Input: part model. Units: mm. Frame: model coordinates. A direction names the side the tool comes from. Give positions to 0.01 mm unless a question says otherwise; leave off trailing zeros. Loops run counter-clockwise (first coordinate to the right, second up) from the corner with the lowest first, then second, coordinate; pieces in that order, holes last. Notation, with made-up numbers: (17, 64.5) -> (71, 64.5) arc R36 ccw to (71, 98.5) -> close; hole circle Ø11 at (-31.75, 3.25). An arc over 180 degrees is marked (long way). One line per question, with ' | ' between items.
from build123d import *

# Parameters (mm, degrees)
SKETCH2_R               = 14
SKETCH2_R_2             = 10
EXTRUDE1_DEPTH          = 25.5
EXTRUDE2_DEPTH          = 10
SKETCH4_W               = 51
SKETCH4_H               = 51
EXTRUDE3_DEPTH          = 3
SKETCH5_W               = 51
SKETCH5_H               = 51
SKETCH5_W_2             = 43
SKETCH5_H_2             = 43
EXTRUDE4_DEPTH          = 40
SKETCH8_W               = 25
SKETCH8_H               = 20
EXTRUDE8_DEPTH          = 40
SKETCH10_W              = 43
SKETCH10_H              = 43
EXTRUDE10_DEPTH         = 45
SKETCH11_R              = 15
EXTRUDE11_DEPTH         = 5
SKETCH12_W              = 5
SKETCH12_H              = 25
EXTRUDE12_DEPTH         = 5
SKETCH13_R              = 1.5
EXTRUDE13_DEPTH         = 5
SKETCH14_R              = 7.5
EXTRUDE14_DEPTH         = 10
SKETCH15_R              = 12.5
EXTRUDE15_DEPTH         = 30
SKETCH16_R              = 5
EXTRUDE16_DEPTH         = 125
EXTRUDE17_START         = 80.797218397
EXTRUDE17_OUTLINE_R     = 12.5
EXTRUDE17_OUTLINE_R_2   = 11.5
EXTRUDE17_DEPTH         = 3.587847701
EXTRUDE17_START_2       = 86.797218397
EXTRUDE17_2_OUTLINE_R   = 12.5
EXTRUDE17_2_OUTLINE_R_2 = 11.5
EXTRUDE17_2_DEPTH       = 3.587847701
EXTRUDE17_START_3       = 92.797218397
EXTRUDE17_3_OUTLINE_R   = 12.5
EXTRUDE17_3_OUTLINE_R_2 = 11.5
EXTRUDE17_3_DEPTH       = 3.587847701
EXTRUDE17_START_4       = 98.797218397
EXTRUDE17_4_OUTLINE_R   = 12.5
EXTRUDE17_4_OUTLINE_R_2 = 11.5
EXTRUDE17_4_DEPTH       = 3.587847701


# Read off the part's stored shape, not the designer's step: Extrude17
with BuildPart() as part:
    # Sketch2 → Extrude1 (new, symmetric)
    with BuildSketch(Plane.XY):
        Circle(SKETCH2_R)
        Circle(SKETCH2_R_2, mode=Mode.SUBTRACT)
    extrude(amount=EXTRUDE1_DEPTH, both=True)

    # Sketch3 → Extrude2 (add, symmetric)
    with BuildSketch(Plane.XY):
        with BuildLine():
            Line((0, 14), (15, 14))
            Line((15, 14), (15, -14))
            Line((15, -14), (0, -14))
            ThreePointArc((0, -14), (14, 0), (0, 14))
        make_face()
    extrude(amount=EXTRUDE2_DEPTH, both=True)

    # Sketch4 → Extrude3 (add)
    with BuildSketch(Plane(origin=(15, 0, 0), x_dir=(0, 0, -1), z_dir=(1, 0, 0))):
        Rectangle(SKETCH4_W, SKETCH4_H)
    extrude(amount=EXTRUDE3_DEPTH)

    # Sketch5 → Extrude4 (add)
    with BuildSketch(Plane(origin=(18, 0, 0), x_dir=(0, 0, -1), z_dir=(1, 0, 0))):
        Rectangle(SKETCH5_W, SKETCH5_H)
        Rectangle(SKETCH5_W_2, SKETCH5_H_2, mode=Mode.SUBTRACT)
    extrude(amount=EXTRUDE4_DEPTH)

    # Sketch8 → Extrude8 (cut)
    with BuildSketch(Plane(origin=(58, 0, 0), x_dir=(0, 0, -1), z_dir=(1, 0, 0))):
        with Locations((0, -25.5)):
            Rectangle(SKETCH8_W, SKETCH8_H)
    extrude(amount=-EXTRUDE8_DEPTH, mode=Mode.SUBTRACT)

    # Sketch10 → Extrude10 (add)
    with BuildSketch(Plane(origin=(18, 0, 0), x_dir=(0, 0, -1), z_dir=(1, 0, 0))):
        Rectangle(SKETCH10_W, SKETCH10_H)
    extrude(amount=EXTRUDE10_DEPTH)

    # Sketch11 → Extrude11 (add)
    with BuildSketch(Plane(origin=(63, 0, 0), x_dir=(0, 0, -1), z_dir=(1, 0, 0))):
        Circle(SKETCH11_R)
    extrude(amount=EXTRUDE11_DEPTH)

    # Sketch12 → Extrude12 (add)
    with BuildSketch(Plane.XZ.offset(21.5)):
        with Locations((20.5, 0)):
            Rectangle(SKETCH12_W, SKETCH12_H)
    extrude(amount=EXTRUDE12_DEPTH)

    # Sketch13 → Extrude13 (add)
    with BuildSketch(Plane.XZ.offset(26.5)):
        with Locations(Location((20.514171065, 8.5, 0), (0, 0, 270))):
            Circle(SKETCH13_R)
        with Locations(Location((20.514171065, 3.5, 0), (0, 0, 270))):
            Circle(SKETCH13_R)
        with Locations(Location((20.514171065, -3.5, 0), (0, 0, 270))):
            Circle(SKETCH13_R)
        with Locations(Location((20.514171065, -8.5, 0), (0, 0, 270))):
            Circle(SKETCH13_R)
    extrude(amount=EXTRUDE13_DEPTH)

    # Sketch14 → Extrude14 (add)
    with BuildSketch(Plane(origin=(68, 0, 0), x_dir=(0, 0, -1), z_dir=(1, 0, 0))):
        Circle(SKETCH14_R)
    extrude(amount=EXTRUDE14_DEPTH)

    # Sketch15 → Extrude15 (add)
    with BuildSketch(Plane(origin=(78, 0, 0), x_dir=(0, 0, -1), z_dir=(1, 0, 0))):
        Circle(SKETCH15_R)
    extrude(amount=EXTRUDE15_DEPTH)

    # Sketch16 → Extrude16 (add)
    with BuildSketch(Plane(origin=(108, 0, 0), x_dir=(0, 0, -1), z_dir=(1, 0, 0))):
        Circle(SKETCH16_R)
    extrude(amount=EXTRUDE16_DEPTH)

    # Extrude17 outline → Extrude17 (cut)
    with BuildSketch(Plane.YZ.offset(EXTRUDE17_START)):
        Circle(EXTRUDE17_OUTLINE_R)
        Circle(EXTRUDE17_OUTLINE_R_2, mode=Mode.SUBTRACT)
    extrude(amount=EXTRUDE17_DEPTH, mode=Mode.SUBTRACT)

    # Extrude17 2 outline → Extrude17 2 (cut)
    with BuildSketch(Plane.YZ.offset(EXTRUDE17_START_2)):
        Circle(EXTRUDE17_2_OUTLINE_R)
        Circle(EXTRUDE17_2_OUTLINE_R_2, mode=Mode.SUBTRACT)
    extrude(amount=EXTRUDE17_2_DEPTH, mode=Mode.SUBTRACT)

    # Extrude17 3 outline → Extrude17 3 (cut)
    with BuildSketch(Plane.YZ.offset(EXTRUDE17_START_3)):
        Circle(EXTRUDE17_3_OUTLINE_R)
        Circle(EXTRUDE17_3_OUTLINE_R_2, mode=Mode.SUBTRACT)
    extrude(amount=EXTRUDE17_3_DEPTH, mode=Mode.SUBTRACT)

    # Extrude17 4 outline → Extrude17 4 (cut)
    with BuildSketch(Plane.YZ.offset(EXTRUDE17_START_4)):
        Circle(EXTRUDE17_4_OUTLINE_R)
        Circle(EXTRUDE17_4_OUTLINE_R_2, mode=Mode.SUBTRACT)
    extrude(amount=EXTRUDE17_4_DEPTH, mode=Mode.SUBTRACT)


solid = part.part
1. Reachability of faces 1 (the cylindrical face through (91.574, -4.788, -11.547)), 2 (the flat face through (60, 21.5, 0)), 3 (the flat face through (92.797, 11, -4)) from +Z, -Z, +X, -X, +Y, -Y: full face, straight path, thin tool, end or side. Return the list, or none.
Determined:
face 1: +X | face 2: +Z, -Z, +X, +Y | face 3: none
2. Pin query (flat end, axial travel): P1, Ø12, axis at x = 7, y = -2, coming from the -Z side; P2, Ø5, axis at x = 74.5, y = 16, coming from the +Z side; P3, Ø1.5, axis at x = 59.5, z = -9.5, coming from the +Y side; P4, Ø2, axis at x = 147.5, y = -4, coming from the -Z side. Return the tip coordinate at first contact, or that it passes through.
Determined:
P1: stops at z = -25.5 | P2: passes through | P3: stops at y = 21.5 | P4: stops at z = -4
3. Ray query, line 1 along Y through (x, z) = (0, 12); line 2 along X through (y, z) = (3.5, -15.5); line 3 along X through (y, z) = (-7, -8). Return the intervals inside material, ascending. Write a range as from..to.
Determined:
line 1: y = -14..-10, 10..14 | line 2: x = -13.56..-9.37, 9.37..13.56, 15..63 | line 3: x = -12.12..-7.14, 7.14..68, 78..108
4. Section query A-A (x = 184). Output: boundary loops of the cut face in (y, z), then the cut area to 3 significant figures.
Determined:
outline: circle Ø10 at (0, 0) | area: 78.5 mm2
5. Pull-direction query (X, two-part tool) for faces 4 (the flat face through (86.797, 11, -4)), 5 (the cylindrical face through (65.465, 0.66, 14.985)); classes: pulls with the +X half, pulls with the -X half, needs draft (parallel to the pull), parting line crosses it, or undercut.
Determined:
face 4: undercut | face 5: needs draft
